Design review of the part built by this model. Coordinates are the model's own, in mm. Face numbers are marked on the shaded views. A direction names the side the tool comes from. Coordinates: 2 decimals unless noted, no trailing zeros. Loops run counter-clockwise (first coordinate to the right, second up) from the corner with the lowest first, then second, coordinate; pieces in that order, holes last. Notation, with made-up numbers: (37.25, -33) -> (41.25, -33) arc R25 ccw to (41.25, -2) -> close; hole circle Ø11 at (31.25, 71). An arc over 180 degrees is marked (long way). Use one line per item in the form item = value. Start each with the question number.
1. Consider section B-B (x = 7.5). State how many separate pieces and enclosed holes the cut face has, then the cut area to 3 significant figures.
2. The part is to be moulded in two halves that separate along Y. For the marked faces 1, 2 and 3, say which applies: released by +Y, released by -Y, zero draft, split by the parting line, or undercut.
3. Consider section A-A (y = 0). State the section outline as (x, z) points (3 decimals), then the cut area to 3 significant figures.
4. Machinability: for the marked faces 4 and 5, which of the approach directions +Z, -Z, +X, -X, +Y, -Y give a long, thin tool a straight path to every point of the face, cutting with its end or side? Answer none if there is none.
5. Wall thickness on line 1 (X direction, y = -13.5, z = 3.25); line 2 (X direction, y = -8, z = 1.25); line 3 (X direction, y = 8, z = 6): over which ranges is each line inside the solid? List them lowest first. Write a range as from..to.
6. For pin 1 (1.6 mm diameter, centred on y = 15.5, z = 2, fed in from -X); pin 2 (2 mm diameter, centred on y = 16, z = 3, fed in from +X); pin 3 (8 mm diameter, centred on x = 10, y = 21, fed in from -Z), all flat-tipped, find the tip position at first contact; note any pin that passes through.
7. Consider section D-D (y = 20). State the section outline as (x, z) points, then the cut area to 3 significant figures.
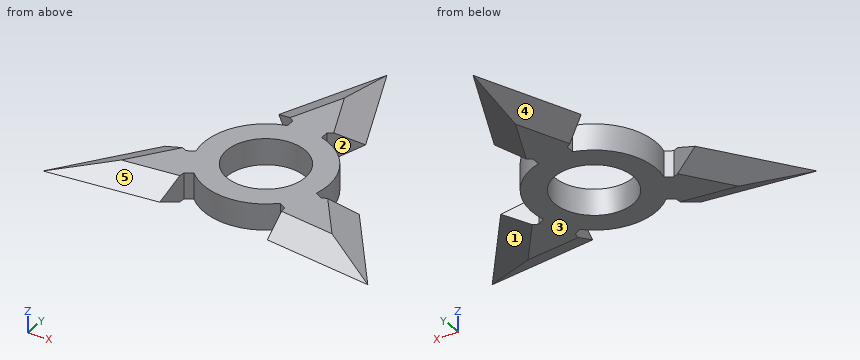
from build123d import *

# Parameters (mm, degrees)
F0_R            = 15.08125
F0_R_2          = 9.525
F1_DEPTH        = 6.35
F3_DEPTH        = 6.35
F3_COPIES_COUNT = 3
F4_SIZE2        = 3.175
F4_SIZE         = 6.35
F4_2_SIZE2      = 3.17499
F4_2_SIZE       = 6.34999


# Not quite as in the source:
# - a fillet or chamfer is up to 0.001 mm smaller than in the source, because OpenCascade refuses the exact size
# - a pattern or mirror of a feature is missing from the dataset's text; its kind, count and spacing are read off the source's solid


with BuildPart() as f1:
    # F0 (on Top) → F1 (new body)
    with BuildSketch(Plane.XY):
        Circle(F0_R)
        Circle(F0_R_2, mode=Mode.SUBTRACT)
    extrude(amount=F1_DEPTH)

    # F2 (on Top) → F3 (join, through all)
    with BuildSketch(Plane.XY):
        with BuildLine():
            Line((10.532929562, 21.1518518627), (0, 45.5084554851))
            Line((0, 45.5084554851), (-10.532929562, 21.1518518627))
            Line((-10.532929562, 21.1518518627), (-4.1548195295, 16.4949237317))
            Line((-4.1548195295, 16.4949237317), (-4.1548195295, 14.497640368))
            ThreePointArc((-4.1548195295, 14.497640368), (0, 15.08125), (4.1548195295, 14.497640368))
            Line((4.1548195295, 14.497640368), (4.1548195295, 16.4949237317))
            Line((4.1548195295, 16.4949237317), (10.532929562, 21.1518518627))
        make_face()
    f3 = extrude(amount=F3_DEPTH)

    # F3_copies: F3 ×3 about axis
    f3_copies_axis = Axis((0, 0, 0), (0, 0, 1))
    for i in range(1, F3_COPIES_COUNT):
        add(f3.rotate(f3_copies_axis, i * 360 / F3_COPIES_COUNT))

    # F4
    f4_edges = [f1.edges().sort_by_distance(p)[0] for p in [
        (-5.266465, 33.330154, 0),
        (5.266465, 33.330154, 0),
        (-31.497992, -12.104185, 0),
        (-26.231527, -21.225969, 0),
        (26.231527, -21.225969, 0),
        (31.497992, -12.104185, 0),
    ]]
    f4_side = f1.faces().sort_by_distance((3.11209, 15.496282, 0))[0]
    chamfer(f4_edges, length=F4_SIZE, length2=F4_SIZE2, reference=f4_side)

    # F4#2 (size 6.35 and 3.175 in the source; OpenCascade refuses exactly that, so slightly less here)
    f4_2_edges = [f1.edges().sort_by_distance(p)[0] for p in [
        (-5.266465, 33.330154, 6.35),
        (5.266465, 33.330154, 6.35),
        (-31.497992, -12.104185, 6.35),
        (-26.231527, -21.225969, 6.35),
        (26.231527, -21.225969, 6.35),
        (31.497992, -12.104185, 6.35),
    ]]
    f4_2_side = f1.faces().sort_by_distance((12.157715, 7.01926, 6.35))[0]
    chamfer(f4_2_edges, length=F4_2_SIZE, length2=F4_2_SIZE2, reference=f4_2_side)


solid = f1.part
Geometry check:
q1.separate_pieces = 3
q1.enclosed_holes = 0
q1.area = 108 mm²
q2.face_1 = released by +Y
q2.face_2 = undercut
q2.face_3 = zero draft
q3.outline = (-15.081, 0) -> (-9.525, 0) -> (-9.525, 6.35) -> (-15.081, 6.35) -> close; (9.525, 0) -> (15.081, 0) -> (15.081, 6.35) -> (9.525, 6.35) -> close
q3.area = 70.6 mm²
q4.face_4 = -Z, -X, +Y
q4.face_5 = +Z, -Y
q5.line_1 = -32.35..-12.39, -6.72..6.72, 12.39..32.35
q5.line_2 = -23.65..-5.17, 5.17..23.65
q5.line_3 = -12.78..-5.17, 5.17..12.78
q6.pin_1 = -4.15
q6.pin_2 = 4.85
q6.pin_3 = 0.9
q7.outline = (-8.96, 2.22) -> (-4.11, 0) -> (4.11, 0) -> (8.96, 2.22) -> (8.96, 4.13) -> (4.11, 6.35) -> (-4.11, 6.35) -> (-8.96, 4.13) -> close
q7.area = 92.2 mm²
